from build123d import *

# Parameters (mm, degrees)
BOSS_EXTRU_1_DEPTH      = 2
ESQUISSE3_R             = 1.5
ESQUISSE3_R_2           = 1.75
ENL_V_MAT_EXTRU_1_DEPTH = 213.141462237
ESQUISSE4_R             = 2
GOUJON_M4X12_DEPTH      = 12


with BuildPart() as part:
    # Esquisse2 → Boss.-Extru.1 (new body)
    with BuildSketch(Plane(origin=(0, 0, 0), x_dir=(1, 0, 0), z_dir=(0, 1, 0))):
        with BuildLine():
            Line((-74.833147735, 130), (74.833147735, 130))
            ThreePointArc((74.833147735, 130), (0, -150), (-74.833147735, 130))
        make_face()
    extrude(amount=BOSS_EXTRU_1_DEPTH)

    # Esquisse3 → Enl_v. mat.-Extru.1 (cut, through all)
    with BuildSketch(Plane(origin=(0, 0, 0), x_dir=(-1, 0, 0), z_dir=(0, -1, 0))):
        with Locations(Location((25, -10, 0), (0, 0, 90))):
            Circle(ESQUISSE3_R)
        with Locations(Location((57, -57, 0), (0, 0, 90))):
            Circle(ESQUISSE3_R)
        with Locations(Location((0, 40, 0), (0, 0, 90))):
            Circle(ESQUISSE3_R_2)
        with Locations(Location((0, 58, 0), (0, 0, 90))):
            Circle(ESQUISSE3_R_2)
        with Locations(Location((-11, 107, 0), (0, 0, 90))):
            Circle(ESQUISSE3_R_2)
        with Locations(Location((11, 85, 0), (0, 0, 90))):
            Circle(ESQUISSE3_R_2)
        with BuildLine():
            Line((125, -20), (125, 20))
            ThreePointArc((125, 20), (133, 28), (141, 20))
            Line((141, 20), (141, -20))
            ThreePointArc((141, -20), (133, -28), (125, -20))
        make_face()
        with BuildLine():
            Line((-141, -20), (-141, 20))
            ThreePointArc((-141, 20), (-133, 28), (-125, 20))
            Line((-125, 20), (-125, -20))
            ThreePointArc((-125, -20), (-133, -28), (-141, -20))
        make_face()
    extrude(amount=-ENL_V_MAT_EXTRU_1_DEPTH, mode=Mode.SUBTRACT)

    # Esquisse4 → Goujon M4x12 (add)
    with BuildSketch(Plane(origin=(0, 2, 0), x_dir=(1, 0, 0), z_dir=(0, 1, 0))):
        with Locations(Location((-100, 60, 0), (0, 0, 270))):
            Circle(ESQUISSE4_R)
    extrude(amount=GOUJON_M4X12_DEPTH)


solid = part.part
Source: CAD feature listing. Evaluate the final solid. Frame: model axes, mm. A direction names the side the tool comes from. Coordinates: 2 decimals unless noted, no trailing zeros. Loops run counter-clockwise (first coordinate to the right, second up) from the corner with the lowest first, then second, coordinate; pieces in that order, holes last. Notation, with made-up numbers: (28.5, -3) - (32.5, -3) arc R26 cw to (32.5, 12) - close; hole circle Ø11 at (37, -12). An arc over 180 degrees is marked (long way). Return JSON: item names as keys, results as strings.
Q1. Section B-B, the plane y = 6.25. Return loops of the section in (x, z).
Results:
{"outline": "circle Ø4 at (-100, -60)"}
Q2. Material intervals for line 1 along Y through (x, z) = (103, -74.5); line 2 along X through (y, z) = (1.4, 10); line 3 along X through (y, z) = (0.7, -107), sorted ascending.
Results:
{"line 1": "0 to 2", "line 2": "-149.67 to -141, -125 to -26.5, -23.5 to 125, 141 to 149.67", "line 3": "-105.12 to 9.25, 12.75 to 105.12"}
Q3. Access query for faces 4 (the flat face through (2, 0, 8)), 5 (the cylindrical face through (133, 1, -28)). Directions: +Z, -Z, +X, -X, +Y, -Y. A direction counts if a zero-diameter tool reaches every point of the face in a straight line with its end or side. Return the directions, or none.
Results:
{"face 4": "+Z, -Z, +X, -X, -Y", "face 5": "+Y, -Y"}
Q4. Section C-C, the plane z = 97.5. Return loops of the section in (x, y).
Results:
{"outline": "(-113.99, 0) - (113.99, 0) - (113.99, 2) - (-113.99, 2) - close"}
Q5. Section D-D, the plane x = 18.5. Return loops of the section in (y, z), plus the area to 3 significant figures.
Results:
{"outline": "(0, -130) - (2, -130) - (2, 148.85) - (0, 148.85) - close", "area": "558 mm2"}
Q6. Section A-A, the plane x = 133. Return loops of the section in (y, z), plus the area to 3 significant figures.
Results:
{"outline": "(0, -69.36) - (2, -69.36) - (2, -28) - (0, -28) - close; (0, 28) - (2, 28) - (2, 69.36) - (0, 69.36) - close", "area": "165 mm2"}
Q7. Mould query, pull axis X, two halves, no side actions, for faces 1 (the cylindrical face through (-133, 1, 28)), 2 (the flat face through (2, 2, 8)), 3 (the cylindrical face through (5.5, 1, 149.9)). Classes: released by +X, released by -X, zero draft, split by the parting line, or undercut.
Results:
{"face 1": "undercut", "face 2": "zero draft", "face 3": "split by the parting line"}
Q8. Contact query for flat-ended pins moving along their axis: P1, Ø4.5, axis at x = 11, z = -107, coming from the -Y side; P2, Ø5, axis at x = -25, z = 10, coming from the +Y side; P3, Ø2, axis at y = 1, z = 5.5, coming from the +X side; P4, Ø2, axis at y = 1.5, z = -6, coming from the -X side. Output: stop coordinate, or through.
Results:
{"P1": "y = 0", "P2": "y = 2", "P3": "x = 149.93", "P4": "x = -149.92"}
